from build123d import *

# Parameters (mm, degrees)
BLANKSKE_W               = 26
BLANKSKE_H               = 4.7
BLANK_DEPTH              = 1
TOOTHCUTSIM_DEPTH        = 27.440310134
TEETHCUTS_COUNT          = 13
TEETHCUTS_PITCH          = 2.199114855
SKETCH3_W                = 17.77574145
SKETCH3_H                = 1
BOSS_EXTRUDE2_DEPTH      = 37
BOSS_EXTRUDE3_DEPTH      = 16
BOSS_EXTRUDE3_DEPTH_BACK = 25.775741
SKETCH4_W                = 1
SKETCH4_H                = 1


with BuildPart() as part:
    # BlankSke → Blank (new body)
    with BuildSketch(Plane.XY):
        with Locations((13, 2.35)):
            Rectangle(BLANKSKE_W, BLANKSKE_H)
    extrude(amount=-BLANK_DEPTH)

    # TooCutSkeSim → ToothCutSim (cut, through all)
    with BuildSketch(Plane.XY):
        Polygon((0.312304759, 3.125), (-0.312304759, 3.125), (-0.894802722, 4.7254), (0.894802722, 4.7254), align=None)
    toothcutsim = extrude(amount=-TOOTHCUTSIM_DEPTH, mode=Mode.SUBTRACT)

    # TeethCuts: ToothCutSim ×13
    with Locations(*[(i * TEETHCUTS_PITCH, 0, 0) for i in range(1, TEETHCUTS_COUNT)]):
        add(toothcutsim, mode=Mode.SUBTRACT)

    # Sketch3 → Boss-Extrude2 (add)
    with BuildSketch(Plane.XZ):
        with Locations((4.112129275, -0.5)):
            Rectangle(SKETCH3_W, SKETCH3_H)
    extrude(amount=BOSS_EXTRUDE2_DEPTH)

    # Sketch4 → Boss-Extrude3 (add, two sides: drawn at the far end of the back side and taken through both)
    with BuildSketch(Plane(origin=(13, 0, 0), x_dir=(0, 0, -1), z_dir=(1, 0, 0)).offset(-BOSS_EXTRUDE3_DEPTH_BACK)):
        with Locations((0.5, -36.5)):
            Rectangle(SKETCH4_W, SKETCH4_H)
    extrude(amount=BOSS_EXTRUDE3_DEPTH + BOSS_EXTRUDE3_DEPTH_BACK)


solid = part.part
Geometry check sheet. Reference: the model listing, model coordinates, mm. A direction names the side the tool comes from. Coordinates: 2 decimals unless noted, no trailing zeros. Loops run counter-clockwise (first coordinate to the right, second up) from the corner with the lowest first, then second, coordinate; pieces in that order, holes last. Notation, with made-up numbers: (-29, 2) - (-17, 2) arc R28 ccw to (-17, 29) - close; hole circle Ø11 at (23, 61.25). An arc over 180 degrees is marked (long way). Use one line per item in the form item = value. Start each with the question number.
Item 1: Thickness scan on probe 1 along Y at (x, z) = (21, -0.5); probe 2 along X at (y, z) = (1.5, -0.9); probe 3 along X at (y, z) = (-1, -0.35). Record the ranges inside material, lowest first.
Item 2: Section check B-B, the plane x = -4. Enter the section's corners in (y, z).
Item 3: Mould release check, pull along X, two halves, no side actions. Record for faces 1 (the face through (8, -16, -1)), 2 (the face through (5, 3.92, -0.49)), 3 (the face through (-4.776, -17.7, -0.5)): +X half, -X half, draft (parallel to the pull), parting line (faces both ways), or undercut.
Item 4: Gauge pin test, flat ends, axial feed: pin 1 (0.5 mm diameter, centred on x = 11, z = -0.5, fed in from +Y) (3 decimals); pin 2 (0.5 mm diameter, centred on y = 1.5, z = -0.5, fed in from -X); pin 3 (0.5 mm diameter, centred on x = 20.5, z = -0.5, fed in from +Y). Record the tip position at first contact, or that the pin passes through.
Item 5: Tool access check on faces 4 (the face through (20.9, -36, -0.5)), 5 (the face through (9.4, 3.92, -0.49)), 6 (the face through (-8.8, -36, -0.5)). Record the directions out of +Z, -Z, +X, -X, +Y, -Y that give a thin tool (end or side, any length) a straight path to the whole face; none if there is none.
Item 6: Section check A-A, the plane y = -13. Enter the section's corners in (x, z), and give its area (3 significant figures).
Computed:
q1.probe_1 = -37 to -36, 0 to 4.7
q1.probe_2 = 0 to 26
q1.probe_3 = -4.78 to 13
q2.outline = (-37, -1) - (0, -1) - (0, 0) - (-37, 0) - close
q3.face_1 = draft
q3.face_2 = undercut
q3.face_3 = -X half
q4.pin_1 = 3.125
q4.pin_2 = 0
q4.pin_3 = 4.7
q5.face_4 = +Z, -Z, +X
q5.face_5 = +Z, -Z, +Y
q5.face_6 = +Z, -Z, -X, +Y
q6.outline = (-4.78, -1) - (13, -1) - (13, 0) - (-4.78, 0) - close
q6.area = 17.8 mm2
